Verification items for this drawing (mm, ordinates from the low corner). A direction names the side the tool comes from. Coordinates: 2 decimals unless noted, no trailing zeros. Order: outer loops, then holes, each group sorted by start corner. A loop starts at its lowest first (then second) coordinate and runs counter-clockwise, first axis right, second up. Notation, with made-up numbers: M -37.75,87.25 L 7.25,87.25 A25 ccw 7.25,123.25 Z; hole C 1,65.5 d11. An arc over 180 degrees is marked long. Return JSON: item names as keys, results as strings. Group by question number.
1. Gauge pin test, flat ends, axial feed: pin 1 (12.5 mm diameter, centred on y = 35, z = 14, fed in from -X); pin 2 (2 mm diameter, centred on x = 8, y = 37, fed in from -Z); pin 3 (2 mm diameter, centred on x = 30, z = 13.5, fed in from +Y); pin 4 (15 mm diameter, centred on x = 25.65, z = 55.95, fed in from -Y). Record the tip position at first contact, or that the pin passes through.
2. Section check D-D, the plane x = 16. Record the cut outline in (y, z) (1 decimal), plus the area to 3 significant figures.
3. Section check A-A, the plane x = 23. Record the cut outline in (y, z).
4. Section check C-C, the plane y = 11. Record the cut outline in (x, z), plus the area to 3 significant figures.
5. Set-up check for the marked faces 5, 6 and 7: record each of +Z, -Z, +X, -X, +Y, -Y from which the full face is reachable in a straight line by a thin tool's end or side.
6. Mould release check, pull along X, two halves, no side actions. Record for the marked faces 1, 2, 3 and 4: +X half, -X half, draft (parallel to the pull), parting line (faces both ways), or undercut.
7. Section check B-B, the plane z = 63. Record the cut outline in (x, y) (1 decimal).
8. Material ranges on line 1 along Z through (x, y) = (39, 32); line 2 along X through (y, z) = (22.5, 18.5); line 3 along X through (y, z) = (6.5, 55), recorded low to high.
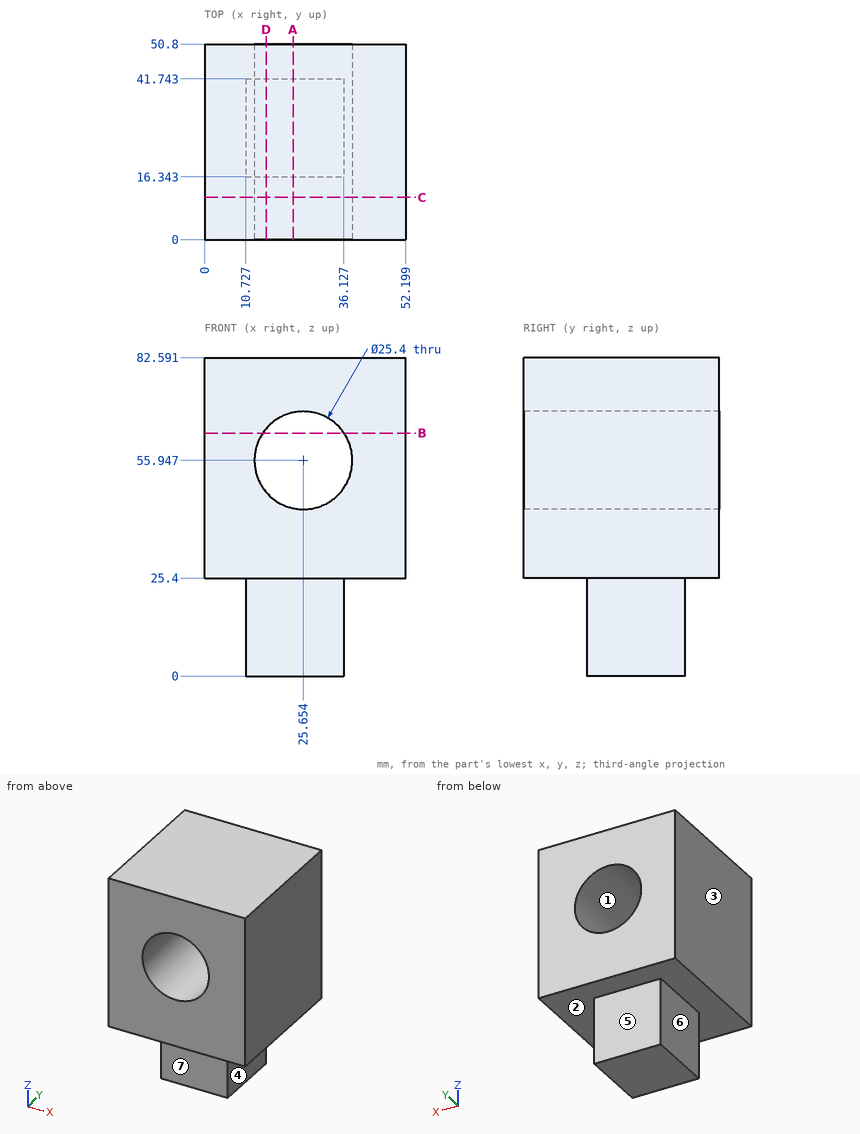
Answers follow:
{
 "1": {"pin 1": "x = 10.73", "pin 2": "z = 25.4", "pin 3": "y = 41.74", "pin 4": "through"},
 "2": {"outline": "M 0,25.4 L 16.3,25.4 L 16.3,0 L 41.7,0 L 41.7,25.4 L 50.8,25.4 L 50.8,47.7 L 0,47.7 Z; M 0,64.2 L 50.8,64.2 L 50.8,82.6 L 0,82.6 Z", "area": "2,710 mm^2"},
 "3": {"outline": "M 0,25.4 L 16.34,25.4 L 16.34,0 L 41.74,0 L 41.74,25.4 L 50.8,25.4 L 50.8,43.53 L 0,43.53 Z; M 0,68.37 L 50.8,68.37 L 50.8,82.59 L 0,82.59 Z"},
 "4": {"outline": "M 0,25.4 L 52.2,25.4 L 52.2,82.59 L 0,82.59 Z; hole C 25.65,55.95 d25.4", "area": "2,480 mm^2"},
 "5": {"face 5": "-Z, +X, -X, +Y", "face 6": "-Z, -X, +Y, -Y", "face 7": "-Z, +X, -X, -Y"},
 "6": {"face 1": "undercut", "face 2": "draft", "face 3": "-X half", "face 4": "+X half"},
 "7": {"outline": "M 0,0 L 15.1,0 L 15.1,50.8 L 0,50.8 Z; M 36.2,0 L 52.2,0 L 52.2,50.8 L 36.2,50.8 Z"},
 "8": {"line 1": "25.4 to 82.59", "line 2": "10.73 to 36.13", "line 3": "0 to 12.99, 38.32 to 52.2"}
}
